Geometry check sheet. Reference: drawing and pictorial views, mm from the part's lowest x, y, z. A direction names the side the tool comes from. Round coordinates to 2 decimals unless told otherwise and drop trailing zeros. Loops run counter-clockwise (first coordinate to the right, second up) from the corner with the lowest first, then second, coordinate; pieces in that order, holes last. Notation, with made-up numbers: M 56,51 L 73,51 A36 ccw 73,90 Z; hole C 62.5,11.25 d3. An arc over 180 degrees is marked long. One line per question, with ' | ' between items. Start each with the question number.
(1) Section check A-A (z = 26). Record the boundary of the cut face in (x, y).
(2) Thickness scan on probe 1 along Z at (x, y) = (40, 11); probe 2 along Y at (x, z) = (56.5, 26.5); probe 3 along Z at (x, y) = (13.5, 37.5). Record the ranges inside material, lowest first. Write a range as [from, to].
(3) Section check B-B (y = 12). Record the boundary of the cut face in (x, z).
(4) Section check C-C (x = 31). Record the boundary of the cut face in (y, z).
(5) Go/stop test with flat-tipped pins: P1, Ø12, axis at x = 15, y = 7, coming from the -Z side; P2, Ø2, axis at x = 43.5, y = 34, coming from the +Z side; P3, Ø11, axis at x = 17.5, y = 12.5, coming from the +Z side; P4, Ø2, axis at x = 32.5, y = 18.5, coming from the +Z side. Record where each tip stops, or that it passes through.
(6) Section check D-D (z = 16.5). Record the boundary of the cut face in (x, y), and give its area (3 significant figures).
(7) Tool access check on the marked faces 1, 2 and 3. Record the directions out of +Z, -Z, +X, -X, +Y, -Y that give a thin tool (end or side, any length) a straight path to the whole face; none if there is none.
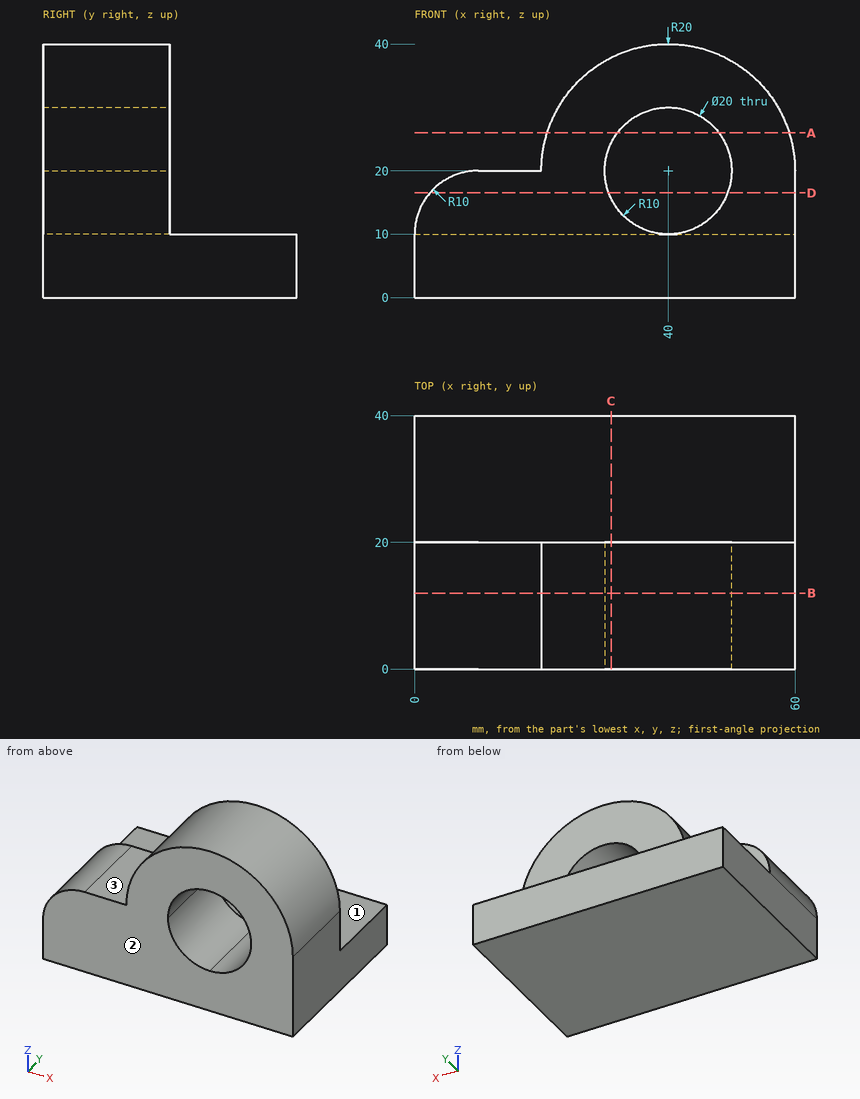
The answers:
1) outline: M 20.92,0 L 32,0 L 32,20 L 20.92,20 Z; M 48,0 L 59.08,0 L 59.08,20 L 48,20 Z
2) probe 1: [0, 10], [30, 40] | probe 2: [0, 20] | probe 3: [0, 10]
3) outline: M 0,0 L 60,0 L 60,20 A20 ccw 20,20 L 10,20 A10 ccw 0,10 Z; hole C 40,20 d20
4) outline: M 0,0 L 40,0 L 40,10 L 20,10 L 20,15.64 L 0,15.64 Z; M 0,24.36 L 20,24.36 L 20,37.86 L 0,37.86 Z
5) P1: z = 0 | P2: z = 10 | P3: z = 30.54 | P4: z = 38.91
6) outline: M 2.4,0 L 30.63,0 L 30.63,20 L 2.4,20 Z; M 49.37,0 L 60,0 L 60,20 L 49.37,20 Z | area: 777 mm²
7) face 1: +Z, +X, -X, +Y | face 2: +Z, -Z, +X, -X, -Y | face 3: +Z, -X, +Y, -Y
